Design review of the part built by this model. Coordinates are the model's own, in mm. Coordinates: 2 decimals unless noted, no trailing zeros. Loops run counter-clockwise (first coordinate to the right, second up) from the corner with the lowest first, then second, coordinate; pieces in that order, holes last.
from build123d import *

# Parameters (mm, degrees)
F0_R          = 9.5
F1_DEPTH      = 630
F2_R          = 6.5
F3_DEPTH      = 25
F3_DEPTH_BACK = 25


with BuildPart() as f1:
    # F0 (on Front) → F1 (new body)
    with BuildSketch(Plane.XZ):
        Circle(F0_R)
    extrude(amount=F1_DEPTH)

    # F2 (on Right) → F3 (cut, two sides)
    with BuildSketch(Plane.YZ) as f3_sk:
        with Locations((-10, 0)):
            Circle(F2_R)
        with Locations((-110, 0)):
            Circle(F2_R)
    extrude(amount=F3_DEPTH, mode=Mode.SUBTRACT)
    extrude(f3_sk.sketch, amount=-F3_DEPTH_BACK, mode=Mode.SUBTRACT)


solid = f1.part
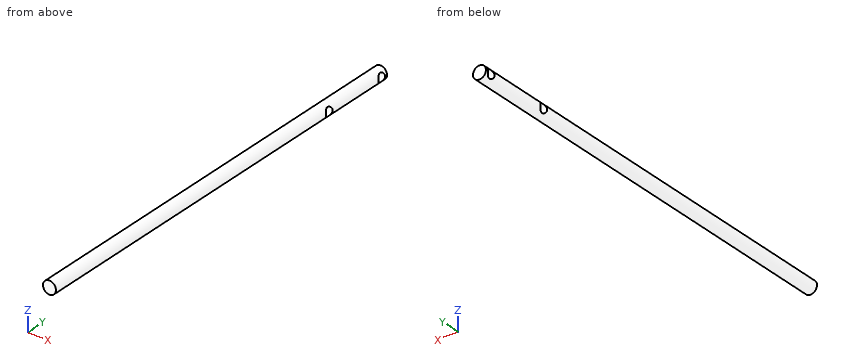
Q1. Take a section at D-D, the plane y = -110. Write out the cut boundary in (x, z), then the cut area to 3 significant figures.
Q2. For line 1 (Y direction, x = -5.25, z = 0); line 2 (Y direction, x = -7.5, z = -1); line 3 (Z direction, x = -0.25, y = -164.5), list the stretches that pass through material, from the lowest coordinate up.
Q3. Take a section at B-B, the plane x = 3. Write out the cut boundary in (y, z).
Q4. Take a section at A-A, the plane z = 0. Write out the cut boundary in (x, y), then the cut area to 3 significant figures.
Q5. Clearance check with flat-ended pins moving along their axes: pin 1 Ø1 at (x, y) = (4.5, -255) entering from +Z; pin 2 Ø5 at (x, y) = (5, -395.5) entering from +Z. State where each tip first meets the part, or that it passes through.
Q6. Take a section at C-C, the plane y = -179. Write out the cut boundary in (x, z).
Entries:
1. outline: (-6.93, -6.5) arc R9.5 ccw to (6.93, -6.5) - close; (-6.93, 6.5) - (6.93, 6.5) arc R9.5 ccw to start
1. area: 57.5 mm2
2. line 1: y = -630 to -116.5, -103.5 to -16.5, -3.5 to 0
2. line 2: y = -630 to -116.42, -103.58 to -16.42, -3.58 to 0
2. line 3: z = -9.5 to 9.5
3. outline: (-630, -9.01) - (0, -9.01) - (0, 9.01) - (-630, 9.01) - close; hole circle Ø13 at (-110, 0); hole circle Ø13 at (-10, 0)
4. outline: (-9.5, -630) - (9.5, -630) - (9.5, -116.5) - (-9.5, -116.5) - close; (-9.5, -103.5) - (9.5, -103.5) - (9.5, -16.5) - (-9.5, -16.5) - close; (-9.5, -3.5) - (9.5, -3.5) - (9.5, 0) - (-9.5, 0) - close
4. area: 11,500 mm2
5. pin 1: stops at z = 8.62
5. pin 2: stops at z = 9.17
6. outline: circle Ø19 at (0, 0)
